```python
from build123d import *

# Parameters (mm, degrees)
SKETCH_1_W          = 34
SKETCH_1_H          = 20
EXTRUDE_1_DEPTH     = 7.5
SKETCH_2_W          = 30
SKETCH_2_H          = 16
CUT_EXTRUDE_1_DEPTH = 5.5
SKETCH_3_W          = 5.5
SKETCH_3_H          = 10
CUT_EXTRUDE_2_DEPTH = 2
SKETCH_4_W          = 5.5
SKETCH_4_H          = 14
CUT_EXTRUDE_3_DEPTH = 2
CUT_EXTRUDE_4_DEPTH = 1.5
SKETCH_6_R          = 1.75
EXTRUDE_2_DEPTH     = 4
SKETCH_7_R          = 0.85
CUT_EXTRUDE_5_DEPTH = 3


with BuildPart() as part:
    # 草图1 → 凸台-拉伸1 (new body)
    with BuildSketch(Plane.XY):
        Rectangle(SKETCH_1_W, SKETCH_1_H)
    extrude(amount=EXTRUDE_1_DEPTH)

    # 草图2 → 切除-拉伸1 (cut)
    with BuildSketch(Plane.XY.offset(7.5)):
        Rectangle(SKETCH_2_W, SKETCH_2_H)
    extrude(amount=-CUT_EXTRUDE_1_DEPTH, mode=Mode.SUBTRACT)

    # 草图3 → 切除-拉伸2 (cut)
    with BuildSketch(Plane(origin=(17, 0, 0), x_dir=(0, 0, -1), z_dir=(1, 0, 0))):
        with Locations((-4.75, 0)):
            Rectangle(SKETCH_3_W, SKETCH_3_H)
    extrude(amount=-CUT_EXTRUDE_2_DEPTH, mode=Mode.SUBTRACT)

    # 草图4 → 切除-拉伸3 (cut)
    with BuildSketch(Plane.ZY.offset(17)):
        with Locations((4.75, 0)):
            Rectangle(SKETCH_4_W, SKETCH_4_H)
    extrude(amount=-CUT_EXTRUDE_3_DEPTH, mode=Mode.SUBTRACT)

    # 草图5 → 切除-拉伸4 (cut)
    with BuildSketch(Plane.XY.offset(7.5)):
        Polygon((-16, 7), (-16, 9), (16, 9), (16, 5), (15, 5), (15, 8), (-15, 8), (-15, 7), align=None)
        Polygon((-15, -7), (-15, -8), (15, -8), (15, -5), (16, -5), (16, -9), (-16, -9), (-16, -7), align=None)
    extrude(amount=-CUT_EXTRUDE_4_DEPTH, mode=Mode.SUBTRACT)

    # 草图6 → 凸台-拉伸2 (add)
    with BuildSketch(Plane.XY.offset(2)):
        with Locations((5, 5)):
            Circle(SKETCH_6_R)
        with Locations((-5, -5)):
            Circle(SKETCH_6_R)
    extrude(amount=EXTRUDE_2_DEPTH)

    # 草图7 → 切除-拉伸5 (cut)
    with BuildSketch(Plane.XY.offset(6)):
        with Locations((-5, -5)):
            Circle(SKETCH_7_R)
        with Locations((5, 5)):
            Circle(SKETCH_7_R)
    extrude(amount=-CUT_EXTRUDE_5_DEPTH, mode=Mode.SUBTRACT)


solid = part.part
```
Input: part model. Units: mm. Frame: model coordinates. A direction names the side the tool comes from. Give positions to 0.01 mm unless a question says otherwise; leave off trailing zeros. Order: outer loops, then holes, each group sorted by start corner. A loop starts at its lowest first (then second) coordinate and runs counter-clockwise, first axis right, second up. Notation, with made-up numbers: (17, -10) - (60, -10) arc R28 cw to (60, 8) - close; hole circle Ø4 at (-20, 70). An arc over 180 degrees is marked (long way). Use a Markdown table: item, result.
(1) Line query: line 1 (Y direction, x = -5, z = 4.55); line 2 (Y direction, x = 5, z = 3.7); line 3 (Y direction, x = 0, z = 6.25). Output: solid intervals per line, ascending. Write a range as from..to.
Computed values:
| item | result |
|---|---|
| line 1 | y = -10..-8, -6.75..-5.85, -4.15..-3.25, 8..10 |
| line 2 | y = -10..-8, 3.25..4.15, 5.85..6.75, 8..10 |
| line 3 | y = -10..-9, 9..10 |
(2) Section query B-B (y = -7.5). Output: boundary loops of the cut face in (x, z), then the cut area to 3 significant figures.
Computed values:
| item | result |
|---|---|
| outline | (-17, 0) - (17, 0) - (17, 7.5) - (16, 7.5) - (16, 6) - (15, 6) - (15, 2) - (-15, 2) - (-15, 6) - (-16, 6) - (-16, 7.5) - (-17, 7.5) - close |
| area | 87.0 mm2 |
(3) Pin query (flat end, axial travel): pin 1 (1.4 mm diameter, centred on x = 5, y = 5, fed in from +Z); pin 2 (3 mm diameter, centred on x = 5.5, y = 5.5, fed in from +Z); pin 3 (1 mm diameter, centred on y = -3, z = 4.5, fed in from +X). Return the tip coordinate at first contact, or that it passes through.
Computed values:
| item | result |
|---|---|
| pin 1 | stops at z = 3 |
| pin 2 | stops at z = 6 |
| pin 3 | stops at x = -4.1 |
(4) Section query A-A (x = -5). Output: boundary loops of the cut face in (y, z), then the cut area to 3 significant figures.
Computed values:
| item | result |
|---|---|
| outline | (-10, 0) - (10, 0) - (10, 7.5) - (9, 7.5) - (9, 6) - (8, 6) - (8, 2) - (-3.25, 2) - (-3.25, 6) - (-4.15, 6) - (-4.15, 3) - (-5.85, 3) - (-5.85, 6) - (-6.75, 6) - (-6.75, 2) - (-8, 2) - (-8, 6) - (-9, 6) - (-9, 7.5) - (-10, 7.5) - close |
| area | 67.9 mm2 |
(5) Section query C-C (x = -1). Output: boundary loops of the cut face in (y, z).
Computed values:
| item | result |
|---|---|
| outline | (-10, 0) - (10, 0) - (10, 7.5) - (9, 7.5) - (9, 6) - (8, 6) - (8, 2) - (-8, 2) - (-8, 6) - (-9, 6) - (-9, 7.5) - (-10, 7.5) - close |
(6) Access query for faces 4 (the flat face through (-15, -7.5, 4)), 5 (the flat face through (5, 4, 6)), 6 (the flat face through (16, -5, 4)). Directions: +Z, -Z, +X, -X, +Y, -Y. A direction counts if a zero-diameter tool reaches every point of the face in a straight line with its end or side. Return the directions, or none.
Computed values:
| item | result |
|---|---|
| face 4 | +Z |
| face 5 | +Z, -X |
| face 6 | +Z, +X |
(7) Draft query along Y for faces 1 (the flat face through (17, 0, 1)), 2 (the flat face through (0, 0, 2)), 3 (the flat face through (0, -10, 4)). Return one class per face: released by +Y, released by -Y, zero draft, split by the parting line, or undercut.
Computed values:
| item | result |
|---|---|
| face 1 | zero draft |
| face 2 | undercut |
| face 3 | released by -Y |
(8) Section query D-D (y = 0). Output: boundary loops of the cut face in (x, z), then the cut area to 3 significant figures.
Computed values:
| item | result |
|---|---|
| outline | (-17, 0) - (17, 0) - (17, 2) - (-17, 2) - close |
| area | 68.0 mm2 |
